Answer from the drawing. Dimensions are ordinates in mm from the lowest x, y and z of the part. A direction names the side the tool comes from. Coordinates: 2 decimals unless noted, no trailing zeros. Write each loop counter-clockwise with the first axis right and the second up, starting at its lowest first coordinate (ties: lowest second). Pieces come first, ordered by that corner, then holes.
1) Find the intervals of material crossed by line 1 (Y direction, x = 6, z = 10.85); line 2 (Y direction, x = 6, z = 5); line 3 (Z direction, x = 10, y = 4.75), in increasing order.
2) Which of the six approach directions +Z, -Z, +X, -X, +Y, -Y give full straight-line access (tool end or side, diameter ignored) to the marked faces 4 and 5?
3) Each of these flat-tipped pins is pushed along its axis until it touches: pin 1 Ø1.5 at (y, z) = (8, 9) entering from +X; pin 2 Ø5 at (x, z) = (6, 4.5) entering from -Y; pin 3 Ø5.5 at (x, y) = (7.5, 7.5) entering from -Z; pin 4 Ø1 at (y, z) = (3, 10.5) entering from +X. Where does it stop, or does it pass through?
4) The part is cut by section D-D (y = 4.75). Determine the outline of the cut face in (x, z).
5) Determine the mould class of the marked faces 1, 2 and 3 for opening direction X: +X half, -X half, draft (parallel to the pull), parting line (faces both ways), or undercut.
6) The part is cut by section A-A (y = 6). Determine the outline of the cut face in (x, z).
7) The part is cut by section B-B (x = 8.5). Determine the outline of the cut face in (y, z).
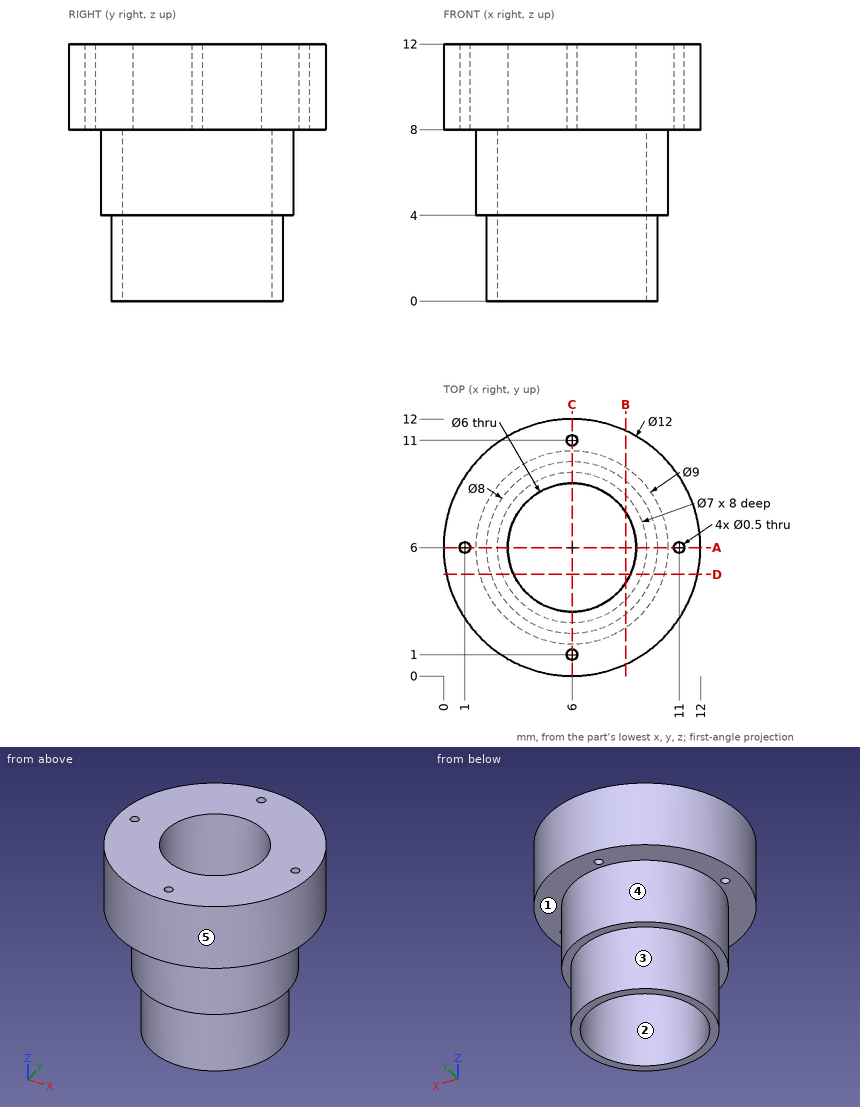
Reported:
1. line 1: y = 0 to 0.75, 1.25 to 3, 9 to 10.75, 11.25 to 12
1. line 2: y = 1.5 to 2.5, 9.5 to 10.5
1. line 3: z = 4 to 12
2. face 4: -Z
2. face 5: +Z, -Z
3. pin 1: stops at x = 11.87
3. pin 2: stops at y = 1.5
3. pin 3: stops at z = 0
3. pin 4: stops at x = 11.45
4. outline: (0.13, 8) - (1.68, 8) - (1.68, 4) - (2.2, 4) - (2.2, 0) - (2.73, 0) - (2.73, 8) - (3.27, 8) - (3.27, 12) - (0.13, 12) - close; (8.73, 8) - (9.27, 8) - (9.27, 0) - (9.8, 0) - (9.8, 4) - (10.32, 4) - (10.32, 8) - (11.87, 8) - (11.87, 12) - (8.73, 12) - close
5. face 1: draft
5. face 2: undercut
5. face 3: parting line
6. outline: (0, 8) - (0.75, 8) - (0.75, 12) - (0, 12) - close; (1.25, 8) - (1.5, 8) - (1.5, 4) - (2, 4) - (2, 0) - (2.5, 0) - (2.5, 8) - (3, 8) - (3, 12) - (1.25, 12) - close; (9, 8) - (9.5, 8) - (9.5, 0) - (10, 0) - (10, 4) - (10.5, 4) - (10.5, 8) - (10.75, 8) - (10.75, 12) - (9, 12) - close; (11.25, 8) - (12, 8) - (12, 12) - (11.25, 12) - close
7. outline: (0.55, 8) - (2.26, 8) - (2.26, 4) - (2.88, 4) - (2.88, 0) - (3.55, 0) - (3.55, 8) - (4.34, 8) - (4.34, 12) - (0.55, 12) - close; (7.66, 8) - (8.45, 8) - (8.45, 0) - (9.12, 0) - (9.12, 4) - (9.74, 4) - (9.74, 8) - (11.45, 8) - (11.45, 12) - (7.66, 12) - close
